Geometry check sheet. Reference: the model listing, model coordinates, mm. A direction names the side the tool comes from. Round coordinates to 2 decimals unless told otherwise and drop trailing zeros. Write each loop counter-clockwise with the first axis right and the second up, starting at its lowest first coordinate (ties: lowest second). Pieces come first, ordered by that corner, then holes. Notation, with made-up numbers: (-35, 51.25) - (-7, 51.25) arc R20 ccw to (-7, 83.25) - close; hole circle Ø7 at (29.25, 33.5). An arc over 180 degrees is marked (long way). Return JSON: item names as keys, results as strings. Group by question number.
Autodesk Inventor part; units mm, degrees
ref_plane "YZ Plane" through (0, 0, 0) normal (1, 0, 0) x (0, 1, 0)
ref_plane "XZ Plane" through (0, 0, 0) normal (0, 1, 0) x (-1, 0, 0)
ref_plane "XY Plane" through (0, 0, 0) normal (0, 0, 1) x (1, 0, 0)
sketch "Sketch1" plane through (0, 0, 0) normal (0, 1, 0) x (-1, 0, 0)
  circle A0 centre (0, 0) radius 2.0955
  dimension "d0" = 4.191
extrude "Extrusion1" add sketch "Sketch1" along normal blind 30.48
sketch "Sketch2" plane through (0, 30.48, 0) normal (0, 1, 0) x (1, 0, 0)
  circle A0 centre (0, 0) radius 3.175
  dimension "d3" = 6.35
extrude "Extrusion2" add sketch "Sketch2" along normal blind 2.54
fillet "Fillet1" radius 3.175 1 edges at (-3.175, 33.02, 0)
thread "Thread1"
properties part number "0.156screw"
1. Depth check by flat-ended pin: pin 1 Ø1.5 at (x, z) = (1.5, -0.5) entering from -Y; pin 2 Ø1 at (x, y) = (0, 26.5) entering from +Z; pin 3 Ø1 at (x, z) = (2, -2.5) entering from -Y. Enter the tip coordinate at first touch or a pass-through.
2. Material ranges on line 1 along Z through (x, y) = (0, 17.5); line 2 along Y through (x, z) = (2.5, 1); line 3 along Y through (x, z) = (-1.25, -2.25), recorded low to high.
3. Section check A-A (y = 17). Enter the section's corners in (x, z), and give its area (3 significant figures).
4. Tool access check on faces 1 (the face through (0, 0, 0)), 2 (the face through (-2, 15.03, -0.63)). Record the directions out of +Z, -Z, +X, -X, +Y, -Y that give a thin tool (end or side, any length) a straight path to the whole face; none if there is none.
Result sheet:
{
 "1": {"pin 1": "stops at y = 0", "pin 2": "stops at z = 2.1", "pin 3": "stops at y = 30.48"},
 "2": {"line 1": "z = -2.1 to 2.1", "line 2": "y = 30.48 to 31.63", "line 3": "y = 30.48 to 31.79"},
 "3": {"outline": "circle Ø4.19 at (0, 0)", "area": "13.8 mm²"},
 "4": {"face 1": "+Z, -Z, +X, -X, -Y", "face 2": "-Y"}
}
